For this review, take the finished solid that the model builds, in its own axes (mm). A direction names the side the tool comes from. Round coordinates to 2 decimals unless told otherwise and drop trailing zeros. Order: outer loops, then holes, each group sorted by start corner. A loop starts at its lowest first (then second) coordinate and runs counter-clockwise, first axis right, second up. Notation, with made-up numbers: (86, -23.75) -> (143, -23.75) arc R14 cw to (143, -17.75) -> close; hole circle Ø6 at (-21, 34.25). An arc over 180 degrees is marked (long way). Put each result on its own line as item: value. Start each with the question number.
```python
from build123d import *

# Parameters (mm, degrees)
SALIENTE_EXTRUIR1_DEPTH = 50
CROQUIS2_W              = 41
CROQUIS2_H              = 41
CORTAR_EXTRUIR1_DEPTH   = 11
CROQUIS3_R              = 1.7
CROQUIS3_R_2            = 19
CORTAR_EXTRUIR2_DEPTH   = 11


with BuildPart() as part:
    # Croquis1 → Saliente-Extruir1 (new body)
    with BuildSketch(Plane.XY):
        with BuildLine():
            Line((8.375, -25), (-8.375, -25))
            Line((-8.375, -25), (-8.375, 25))
            Line((-8.375, 25), (8.375, 25))
            ThreePointArc((8.375, 25), (2.389225586, 0), (8.375, -25))
        make_face()
    extrude(amount=SALIENTE_EXTRUIR1_DEPTH)

    # Croquis2 → Cortar-Extruir1 (cut)
    with BuildSketch(Plane.ZY.offset(8.375)):
        with Locations((25, 0)):
            Rectangle(CROQUIS2_W, CROQUIS2_H)
    extrude(amount=-CORTAR_EXTRUIR1_DEPTH, mode=Mode.SUBTRACT)

    # Croquis3 → Cortar-Extruir2 (cut)
    with BuildSketch(Plane.ZY.offset(-2.625)):
        with Locations((9, 16)):
            Circle(CROQUIS3_R)
        with Locations((41, 16)):
            Circle(CROQUIS3_R)
        with Locations((41, -16)):
            Circle(CROQUIS3_R)
        with Locations((9, -16)):
            Circle(CROQUIS3_R)
        with Locations((25, 0)):
            Circle(CROQUIS3_R_2)
    extrude(amount=-CORTAR_EXTRUIR2_DEPTH, mode=Mode.SUBTRACT)


solid = part.part
```
Item 1: Consider section A-A, the plane y = -16. Write out the cut boundary in (x, z) (3 decimals), plus the area to 3 significant figures.
Item 2: Insertion check: pin 1 Ø1.5 at (x, y) = (-4, 11) entering from -Z; pin 2 Ø4.5 at (y, z) = (16.5, 24) entering from -X; pin 3 Ø7.5 at (y, z) = (-15.5, 16.5) entering from -X (3 decimals); pin 4 Ø12 at (y, z) = (13, 43.5) entering from +X. Each pin has a flat end and moves straight along its axis. Give the tip position at first contact, or say it passes through.
Item 3: Consider section D-D, the plane y = -4. Write out the cut boundary in (x, z) (3 decimals).
Item 4: Mouldability with a two-part tool opening along Y and no side actions: class faces 4 (the face through (-8.375, -23, 25)), 5 (the face through (3.666, 11.802, 7.983)), 6 (the face through (0, 25, 25)) as +Y half, -Y half, draft (parallel to the pull), parting line (faces both ways), or undercut.
Item 5: Consider section B-B, the plane z = 13. Write out the cut boundary in (x, y) (3 decimals), plus the area to 3 significant figures.
Item 6: Tool access review of faces 1 (the face through (-3, 20.5, 25)), 2 (the face through (4, 19, 25)), 3 (the face through (0, -25, 25)): name each direction out of +Z, -Z, +X, -X, +Y, -Y from which nothing blocks a thin tool from reaching the whole face with its end or side.
Item 7: For L1, parallel to Y at x = 1, z = 6.5; L2, parallel to Z at x = 4.45, y = -16; L3, parallel to Z at x = -4.25, y = 6, list the stretches that pass through material, from the lowest coordinate up.
Item 8: Consider section C-C, the plane x = 0. Write out the cut boundary in (y, z).
Evaluation:
1. outline: (-8.375, 0) -> (4.759, 0) -> (4.759, 7.3) -> (2.625, 7.3) -> (2.625, 4.5) -> (-8.375, 4.5) -> close; (-8.375, 45.5) -> (2.625, 45.5) -> (2.625, 42.7) -> (4.759, 42.7) -> (4.759, 50) -> (-8.375, 50) -> close; (2.625, 10.7) -> (4.759, 10.7) -> (4.759, 14.753) -> (2.625, 14.753) -> close; (2.625, 35.247) -> (4.759, 35.247) -> (4.759, 39.3) -> (2.625, 39.3) -> close
1. area: 147 mm^2
2. pin 1: stops at z = 0
2. pin 2: passes through
2. pin 3: stops at x = 2.625
2. pin 4: stops at x = 5.76
3. outline: (-8.375, 0) -> (2.534, 0) -> (2.534, 4.5) -> (-8.375, 4.5) -> close; (-8.375, 45.5) -> (2.534, 45.5) -> (2.534, 50) -> (-8.375, 50) -> close
4. face 4: draft
4. face 5: undercut
4. face 6: +Y half
5. outline: (-8.375, -25) -> (8.375, -25) arc R55.2 cw to (4.391, -14.731) -> (2.625, -14.731) -> (2.625, -20.5) -> (-8.375, -20.5) -> close; (-8.375, 20.5) -> (2.625, 20.5) -> (2.625, 14.731) -> (4.391, 14.731) arc R55.2 cw to (8.375, 25) -> (-8.375, 25) -> close
5. area: 172 mm^2
6. face 1: -X
6. face 2: +X, -X
6. face 3: +Z, -Z, +X, -X, -Y
7. L1: y = -25 to -20.5, 20.5 to 25
7. L2: z = 0 to 7.3, 10.7 to 14.75, 35.25 to 39.3, 42.7 to 50
7. L3: z = 0 to 4.5, 45.5 to 50
8. outline: (-25, 0) -> (25, 0) -> (25, 50) -> (-25, 50) -> close; hole (-20.5, 4.5) -> (20.5, 4.5) -> (20.5, 45.5) -> (-20.5, 45.5) -> close
